```python
from build123d import *
from build123d.topology import SkipClean

# Parameters (mm, degrees)
SKETCH_1_R          = 21
EXTRUDE_1_DEPTH     = 15
EXTRUDE_START       = 6
EXTRUDE_2_DEPTH     = 6
EXTRUDE_3_DEPTH     = 6
EXTRUDE_START_2     = 9
EXTRUDE_4_DEPTH     = 9
SKETCH_6_R          = 11
EXTRUDE_5_DEPTH     = 3
SKETCH_7_R          = 3
EXTRUDE_6_DEPTH     = 14
EXTRUDE_START_3     = -1
SKETCH_8_R          = 2
EXTRUDE_7_DEPTH     = 1
EXTRUDE_START_4     = -11
SKETCH_9_R          = 7
SKETCH_9_R_2        = 3
EXTRUDE_8_DEPTH     = 11
CUT_EXTRUDE_START   = -10
SKETCH_10_R         = 7
SKETCH_10_R_2       = 5.5
CUT_EXTRUDE_1_DEPTH = 10


with BuildPart() as part:
    # 草图1 → 凸台-拉伸1 (new body)
    with BuildSketch(Plane.XY):
        Circle(SKETCH_1_R)
    extrude(amount=EXTRUDE_1_DEPTH)

    # 草图2 → 凸台-拉伸2 (add)
    with SkipClean():  # the faces are left unmerged after this step: merging them gives an invalid solid
        with BuildSketch(Plane(origin=(0, 0, 0), x_dir=(-1, 0, 0), z_dir=(0, 0, -1)).offset(EXTRUDE_START)):
            with BuildLine():
                Line((2.5, 20.850659462), (2.5, 20.346989949))
                ThreePointArc((2.5, 20.346989949), (0, 20.5), (-2.5, 20.346989949))
                Line((-2.5, 20.346989949), (-2.5, 20.850659462))
                ThreePointArc((-2.5, 20.850659462), (-18.186533479, 10.5), (-19.30720078, -8.260266222))
                Line((-19.30720078, -8.260266222), (-18.871010187, -8.008431465))
                ThreePointArc((-18.871010187, -8.008431465), (-17.753520778, -10.25), (-16.371010187, -12.338558484))
                Line((-16.371010187, -12.338558484), (-16.80720078, -12.59039324))
                ThreePointArc((-16.80720078, -12.59039324), (-15.938440593, -13.673555187), (-15, -14.696938457))
                Line((-15, -14.696938457), (-15, -13.973188612))
                ThreePointArc((-15, -13.973188612), (0, -20.5), (15, -13.973188612))
                Line((15, -13.973188612), (15, -14.696938457))
                ThreePointArc((15, -14.696938457), (15.938440593, -13.673555187), (16.80720078, -12.59039324))
                Line((16.80720078, -12.59039324), (16.371010187, -12.338558484))
                ThreePointArc((16.371010187, -12.338558484), (17.753520778, -10.25), (18.871010187, -8.008431465))
                Line((18.871010187, -8.008431465), (19.30720078, -8.260266222))
                ThreePointArc((19.30720078, -8.260266222), (18.186533479, 10.5), (2.5, 20.850659462))
            make_face()
        extrude(amount=-EXTRUDE_2_DEPTH)

    # 草图4 → 凸台-拉伸3 (add)
    with SkipClean():  # the faces are left unmerged after this step: merging them gives an invalid solid
        with BuildSketch(Plane(origin=(0, 0, -6), x_dir=(-1, 0, 0), z_dir=(0, 0, -1)).offset(EXTRUDE_START)):
            with BuildLine():
                Line((10, -17.895530168), (10, -24))
                Line((10, -24), (-10, -24))
                Line((-10, -24), (-10, -17.895530168))
                ThreePointArc((-10, -17.895530168), (-12.652912345, -16.129284212), (-15, -13.973188612))
                Line((-15, -13.973188612), (-15, -14.696938457))
                ThreePointArc((-15, -14.696938457), (-15.938440593, -13.673555187), (-16.80720078, -12.59039324))
                Line((-16.80720078, -12.59039324), (-16.371010187, -12.338558484))
                ThreePointArc((-16.371010187, -12.338558484), (-17.753520778, -10.25), (-18.871010187, -8.008431465))
                Line((-18.871010187, -8.008431465), (-19.30720078, -8.260266222))
                ThreePointArc((-19.30720078, -8.260266222), (-18.186533479, 10.5), (-2.5, 20.850659462))
                Line((-2.5, 20.850659462), (-2.5, 20.346989949))
                ThreePointArc((-2.5, 20.346989949), (0, 20.5), (2.5, 20.346989949))
                Line((2.5, 20.346989949), (2.5, 20.850659462))
                ThreePointArc((2.5, 20.850659462), (18.186533479, 10.5), (19.30720078, -8.260266222))
                Line((19.30720078, -8.260266222), (18.871010187, -8.008431465))
                ThreePointArc((18.871010187, -8.008431465), (17.753520778, -10.25), (16.371010187, -12.338558484))
                Line((16.371010187, -12.338558484), (16.80720078, -12.59039324))
                ThreePointArc((16.80720078, -12.59039324), (15.938440593, -13.673555187), (15, -14.696938457))
                Line((15, -14.696938457), (15, -13.973188612))
                ThreePointArc((15, -13.973188612), (12.652912345, -16.129284212), (10, -17.895530168))
            make_face()
        extrude(amount=-EXTRUDE_3_DEPTH)

    # 草图5 → 凸台-拉伸4 (add)
    with SkipClean():  # the faces are left unmerged after this step: merging them gives an invalid solid
        with BuildSketch(Plane(origin=(0, 0, -12), x_dir=(-1, 0, 0), z_dir=(0, 0, -1)).offset(EXTRUDE_START_2)):
            with BuildLine():
                Line((18.871010187, -8.008431465), (19.30720078, -8.260266222))
                ThreePointArc((19.30720078, -8.260266222), (18.186533479, 10.5), (2.5, 20.850659462))
                Line((2.5, 20.850659462), (2.5, 20.346989949))
                ThreePointArc((2.5, 20.346989949), (0, 20.5), (-2.5, 20.346989949))
                Line((-2.5, 20.346989949), (-2.5, 20.850659462))
                ThreePointArc((-2.5, 20.850659462), (-18.186533479, 10.5), (-19.30720078, -8.260266222))
                Line((-19.30720078, -8.260266222), (-18.871010187, -8.008431465))
                ThreePointArc((-18.871010187, -8.008431465), (-17.753520778, -10.25), (-16.371010187, -12.338558484))
                Line((-16.371010187, -12.338558484), (-16.80720078, -12.59039324))
                ThreePointArc((-16.80720078, -12.59039324), (-15.938440593, -13.673555187), (-15, -14.696938457))
                ThreePointArc((-15, -14.696938457), (0, -21), (15, -14.696938457))
                ThreePointArc((15, -14.696938457), (15.938440593, -13.673555187), (16.80720078, -12.59039324))
                Line((16.80720078, -12.59039324), (16.371010187, -12.338558484))
                ThreePointArc((16.371010187, -12.338558484), (17.753520778, -10.25), (18.871010187, -8.008431465))
            make_face()
        extrude(amount=-EXTRUDE_4_DEPTH)

    # 草图6 → 凸台-拉伸5 (add)
    with SkipClean():  # the faces are left unmerged after this step: merging them gives an invalid solid
        with BuildSketch(Plane.XY.offset(15)):
            Circle(SKETCH_6_R)
        extrude(amount=EXTRUDE_5_DEPTH)

    # 草图7 → 凸台-拉伸6 (add)
    with SkipClean():  # the faces are left unmerged after this step: merging them gives an invalid solid
        with BuildSketch(Plane.XY.offset(18)):
            Circle(SKETCH_7_R)
        extrude(amount=EXTRUDE_6_DEPTH)

    # 草图8 → 凸台-拉伸7 (add)
    # profile 1 of 2: a face of its own
    with SkipClean():  # the faces are left unmerged after this step: merging them gives an invalid solid
        with BuildSketch(Plane.XY.offset(15).offset(EXTRUDE_START_3)):
            with BuildLine():
                Line((21.566756826, -15.202795796), (17.68629022, -11.322329189))
                ThreePointArc((17.68629022, -11.322329189), (14.849242405, -14.849242405), (11.322329189, -17.68629022))
                Line((11.322329189, -17.68629022), (15.202795796, -21.566756826))
                ThreePointArc((15.202795796, -21.566756826), (21.566756826, -21.566756826), (21.566756826, -15.202795796))
            make_face()
            with Locations((18.384776311, -18.384776311)):
                Circle(SKETCH_8_R, mode=Mode.SUBTRACT)
        # profile 2 of 2: a face of its own
        with BuildSketch(Plane.XY.offset(15).offset(EXTRUDE_START_3)):
            with BuildLine():
                Line((-11.322329189, 17.68629022), (-15.202795796, 21.566756826))
                ThreePointArc((-15.202795796, 21.566756826), (-21.566756826, 21.566756826), (-21.566756826, 15.202795796))
                Line((-21.566756826, 15.202795796), (-17.68629022, 11.322329189))
                ThreePointArc((-17.68629022, 11.322329189), (-14.849242405, 14.849242405), (-11.322329189, 17.68629022))
            make_face()
            with Locations((-18.384776311, 18.384776311)):
                Circle(SKETCH_8_R, mode=Mode.SUBTRACT)
        extrude(amount=EXTRUDE_7_DEPTH)

    # 草图9 → 凸台-拉伸8 (add)
    with SkipClean():  # the faces are left unmerged after this step: merging them gives an invalid solid
        with BuildSketch(Plane.XY.offset(32).offset(EXTRUDE_START_4)):
            Circle(SKETCH_9_R)
            Circle(SKETCH_9_R_2, mode=Mode.SUBTRACT)
        extrude(amount=EXTRUDE_8_DEPTH)

    # 草图10 → 切除-拉伸1 (cut)
    with SkipClean():  # the faces are left unmerged after this step: merging them gives an invalid solid
        with BuildSketch(Plane.XY.offset(32).offset(CUT_EXTRUDE_START)):
            Circle(SKETCH_10_R)
            Circle(SKETCH_10_R_2, mode=Mode.SUBTRACT)
        extrude(amount=CUT_EXTRUDE_1_DEPTH, mode=Mode.SUBTRACT)


solid = part.part
```
Input: part model. Units: mm. Frame: model coordinates. A direction names the side the tool comes from. Round coordinates to 2 decimals unless told otherwise and drop trailing zeros. Loops run counter-clockwise (first coordinate to the right, second up) from the corner with the lowest first, then second, coordinate; pieces in that order, holes last. Notation, with made-up numbers: M -28,51.5 L 1,51.5 A24 ccw 1,87.5 Z; hole C 82,-2.75 d10. An arc over 180 degrees is marked long. Answer in a Markdown table with one row per item. Add a question column.
1. Contact query for flat-ended pins moving along their axis: pin 1 (1 mm diameter, centred on y = 1, z = 16, fed in from +X); pin 2 (12 mm diameter, centred on y = 11.5, z = 2.5, fed in from +X); pin 3 (12 mm diameter, centred on x = 3.5, z = -3.5, fed in from +Y); pin 4 (2.5 mm diameter, centred on x = 18, y = -10, fed in from -Z). Output: stop coordinate, or through.
2. Section C-C (x = 0). Output: boundary loops of the cut face in (y, z).
3. Section B-B (y = 0). Output: boundary loops of the cut face in (x, z), and give its area (3 significant figures).
4. Section D-D (y = -9). Output: boundary loops of the cut face in (x, z), and give its area (3 significant figures).
5. Ray query, probe 1 along Z at (x, y) = (0, 4.5); probe 2 along Z at (x, y) = (-4, 4); probe 3 along Y at (x, z) = (-14.5, 4.5). Return the intervals inside material, ascending.
6. Mould query, pull axis Y, two halves, no side actions, for faces 4 (the face through (-2.38, -10.74, 16.48)), 5 (the face through (19.654, -13.29, 14.493)), 6 (the face through (10, -21, -9)). Classes: released by +Y, released by -Y, zero draft, split by the parting line, or undercut.
7. Set-up query: faces 1 (the face through (0, 20.5, -10.6)), 2 (the face through (6.466, -2.681, 21.493)), 3 (the face through (13.235, -19.599, 14.493)). Return all of +Z, -Z, +X, -X, +Y, -Y with unobstructed straight access to the full face (end or side cutting, diameter ignored); none if empty.
8. Section A-A (z = -15.5). Output: boundary loops of the cut face in (x, y), and give its area (3 significant figures).
Values follow:
| question | item | result |
|---|---|---|
| 1 | pin 1 | x = 10.99 |
| 1 | pin 2 | x = 20.27 |
| 1 | pin 3 | y = 21 |
| 1 | pin 4 | z = -21 |
| 2 | outline | M -24,-12 L -21,-12 L -21,-21 L 20.5,-21 L 20.5,0 L 21,0 L 21,15 L 11,15 L 11,18 L 3,18 L 3,21 L 7,21 L 7,22 L 5.5,22 L 5.5,32 L -5.5,32 L -5.5,22 L -7,22 L -7,21 L -3,21 L -3,18 L -11,18 L -11,15 L -21,15 L -21,0 L -20.5,0 L -20.5,-6 L -24,-6 Z |
| 3 | outline | M -21,-21 L 21,-21 L 21,15 L 11,15 L 11,18 L 3,18 L 3,21 L 7,21 L 7,22 L 5.5,22 L 5.5,32 L -5.5,32 L -5.5,22 L -7,22 L -7,21 L -3,21 L -3,18 L -11,18 L -11,15 L -21,15 Z |
| 3 | area | 1,720 mm^2 |
| 4 | outline | M -18.97,0 L -18.42,0 L -18.42,-21 L 18.42,-21 L 18.42,0 L 18.97,0 L 18.97,15 L 6.32,15 L 6.32,18 L -6.32,18 L -6.32,15 L -18.97,15 Z |
| 4 | area | 1,380 mm^2 |
| 5 | probe 1 | -21 to 18, 21 to 32 |
| 5 | probe 2 | -21 to 18, 21 to 22 |
| 5 | probe 3 | -15.19 to 15.19 |
| 6 | face 4 | split by the parting line |
| 6 | face 5 | undercut |
| 6 | face 6 | zero draft |
| 7 | face 1 | -Z, +Y |
| 7 | face 2 | +Z |
| 7 | face 3 | +Z, -Z, -Y |
| 8 | outline | M -19.31,-8.26 L -18.87,-8.01 A20.5 ccw -16.37,-12.34 L -16.81,-12.59 A21 ccw 16.81,-12.59 L 16.37,-12.34 A20.5 ccw 18.87,-8.01 L 19.31,-8.26 A21 ccw 2.5,20.85 L 2.5,20.35 A20.5 ccw -2.5,20.35 L -2.5,20.85 A21 ccw Z |
| 8 | area | 1,380 mm^2 |
